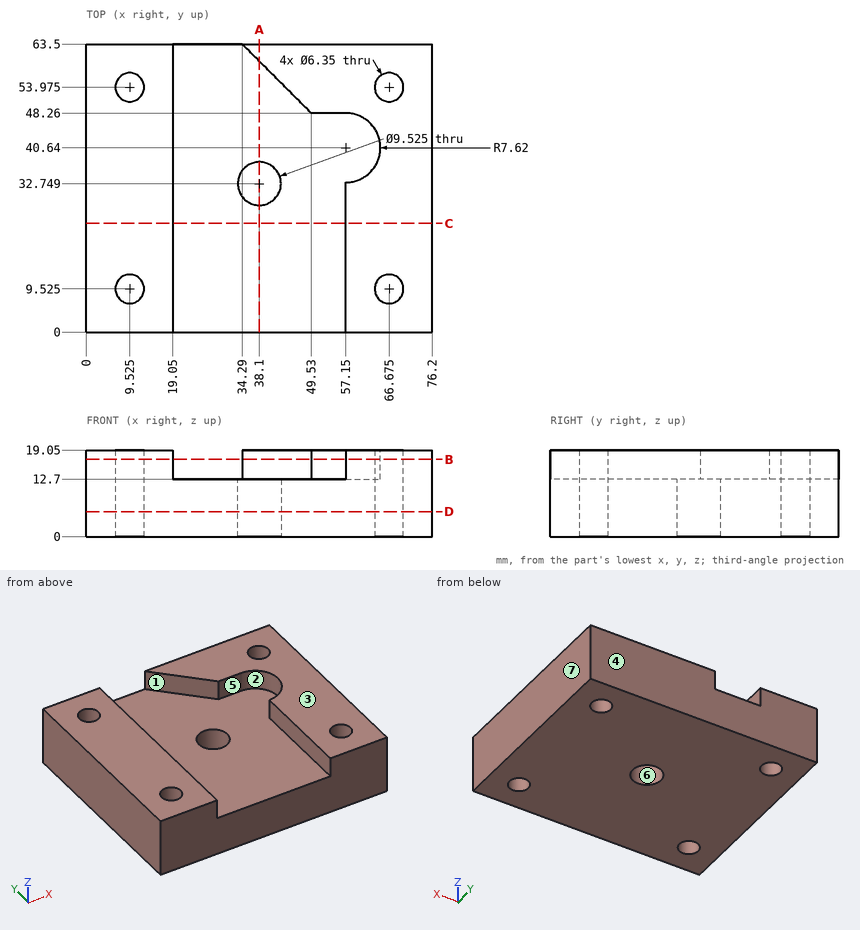
The drawing under review shows one solid part. Ordinate dimensions are in mm from its lowest x, y, z. A direction names the side the tool comes from. Round coordinates to 2 decimals unless told otherwise and drop trailing zeros. Order: outer loops, then holes, each group sorted by start corner. A loop starts at its lowest first (then second) coordinate and runs counter-clockwise, first axis right, second up. Notation, with made-up numbers: (71, 69) -> (97, 69) arc R18 cw to (97, 96) -> close; hole circle Ø6 at (83, 73.5). An arc over 180 degrees is marked (long way). Use a Markdown table: item, result.
Q1. We need section A-A on x = 38.1. Write out the cut boundary in (y, z).
Values:
| item | result |
|---|---|
| outline | (0, 0) -> (27.99, 0) -> (27.99, 12.7) -> (0, 12.7) -> close; (37.51, 0) -> (63.5, 0) -> (63.5, 19.05) -> (59.69, 19.05) -> (59.69, 12.7) -> (37.51, 12.7) -> close |
Q2. Tool access review of the marked faces 1, 2 and 3: name each direction out of +Z, -Z, +X, -X, +Y, -Y from which nothing blocks a thin tool from reaching the whole face with its end or side.
Values:
| item | result |
|---|---|
| face 1 | +Z, -Y |
| face 2 | +Z |
| face 3 | +Z, +X, -X, +Y, -Y |
Q3. We need section D-D on z = 5.5. State how many separate pieces and enclosed holes the cut face has, then the cut area to 3 significant figures.
Values:
| item | result |
|---|---|
| separate pieces | 1 |
| enclosed holes | 5 |
| area | 4,640 mm^2 |
Q4. For line 1 (X direction, y = 9.5, z = 17); line 2 (X direction, y = 54, z = 2); line 3 (X direction, y = 52, z = 12.25), list the stretches that pass through material, from the lowest coordinate up.
Values:
| item | result |
|---|---|
| line 1 | x = 0 to 6.35, 12.7 to 19.05, 57.15 to 63.5, 69.85 to 76.2 |
| line 2 | x = 0 to 6.35, 12.7 to 63.5, 69.85 to 76.2 |
| line 3 | x = 0 to 7.04, 12.01 to 64.19, 69.16 to 76.2 |
Q5. We need section B-B on z = 17. Write out the cut boundary in (x, y) (3 decimals).
Values:
| item | result |
|---|---|
| outline | (0, 0) -> (19.05, 0) -> (19.05, 63.5) -> (0, 63.5) -> close; (34.29, 63.5) -> (49.53, 48.26) -> (57.15, 48.26) arc R7.62 cw to (57.15, 33.02) -> (57.15, 0) -> (76.2, 0) -> (76.2, 63.5) -> close; hole circle Ø6.35 at (9.525, 9.525); hole circle Ø6.35 at (9.525, 53.975); hole circle Ø6.35 at (66.675, 9.525); hole circle Ø6.35 at (66.675, 53.975) |
Q6. We need section C-C on y = 24. Write out the cut boundary in (x, z).
Values:
| item | result |
|---|---|
| outline | (0, 0) -> (76.2, 0) -> (76.2, 19.05) -> (57.15, 19.05) -> (57.15, 12.7) -> (19.05, 12.7) -> (19.05, 19.05) -> (0, 19.05) -> close |
Q7. Mouldability with a two-part tool opening along Y and no side actions: class the marked faces 4, 5, 6 and 7 as +Y half, -Y half, draft (parallel to the pull), parting line (faces both ways), or undercut.
Values:
| item | result |
|---|---|
| face 4 | +Y half |
| face 5 | -Y half |
| face 6 | undercut |
| face 7 | draft |
